```python
from build123d import *

# Parameters (mm, degrees)
SKETCH_1_R          = 2.5
EXTRUDE_1_DEPTH     = 10
SKETCH_2_R          = 2.5
CUT_EXTRUDE_1_DEPTH = 5
SKETCH_3_R          = 2.5
CUT_EXTRUDE_2_DEPTH = 5


with BuildPart() as part:
    # 草图1 → 凸台-拉伸1 (new body)
    with BuildSketch(Plane.XY):
        with BuildLine():
            Line((5, 0), (15, 0))
            Line((15, 0), (15, -5))
            Line((15, -5), (-15, -5))
            Line((-15, -5), (-15, 0))
            Line((-15, 0), (-5, 0))
            Line((-5, 0), (-5, 6))
            ThreePointArc((-5, 6), (0, 11), (5, 6))
            Line((5, 6), (5, 0))
        make_face()
        with Locations((0, 6)):
            Circle(SKETCH_1_R, mode=Mode.SUBTRACT)
    extrude(amount=EXTRUDE_1_DEPTH)

    # 草图2 → 切除-拉伸1 (cut)
    with BuildSketch(Plane(origin=(0, 0, 0), x_dir=(1, 0, 0), z_dir=(0, 1, 0))):
        with Locations(Location((-10, -5, 0), (0, 0, 180))):
            Circle(SKETCH_2_R)
    extrude(amount=-CUT_EXTRUDE_1_DEPTH, mode=Mode.SUBTRACT)

    # 草图3 → 切除-拉伸2 (cut)
    with BuildSketch(Plane(origin=(0, 0, 0), x_dir=(1, 0, 0), z_dir=(0, 1, 0))):
        with Locations(Location((10, -5, 0), (0, 0, 180))):
            Circle(SKETCH_3_R)
    extrude(amount=-CUT_EXTRUDE_2_DEPTH, mode=Mode.SUBTRACT)


solid = part.part
```
The model under review builds one solid part; all positions refer to its coordinate system, in mm. A direction names the side the tool comes from. Coordinates: 2 decimals unless noted, no trailing zeros. Write each loop counter-clockwise with the first axis right and the second up, starting at its lowest first coordinate (ties: lowest second). Pieces come first, ordered by that corner, then holes.
1) To check wall thickness, follow probe 1 along Z at (x, y) = (-10, -2.5); probe 2 along X at (y, z) = (-0.5, 4); probe 3 along Y at (x, z) = (0, 6.5). State the ranges of each line that lie inside material, in increasing order.
2) We need section D-D on y = 6.5. State the section outline as (x, z) points.
3) Clearance check with flat-ended pins moving along their axes: pin 1 Ø5 at (x, z) = (-12, 6) entering from +Y; pin 2 Ø1.8 at (y, z) = (3.5, 5) entering from +X; pin 3 Ø3 at (x, y) = (0, 6) entering from +Z. State where each tip first meets the part, or that it passes through.
4) We need section C-C on z = 1.75. State the section outline as (x, y) points.
5) We need section A-A on z = 3. State the section outline as (x, y) points.
6) We need section B-B on x = -10. State the section outline as (y, z) points, then the cut area to 3 significant figures.
7) Machinability: for faces 1 (the face through (-5, 3, 5)), 2 (the face through (-0.33, 8.48, 4.93)), which of the approach directions +Z, -Z, +X, -X, +Y, -Y give a long, thin tool a straight path to every point of the face, cutting with its end or side? Answer none if there is none.
8) The part is to be moulded in two halves that separate along X. For faces 3 (the face through (-9.67, -2.46, 7.48)), 4 (the face through (8, 0, 3)), 5 (the face through (5, 3, 5)), say which applies: pulls with the +X half, pulls with the -X half, needs draft (parallel to the pull), parting line crosses it, or undercut.
Answer list:
1. probe 1: z = 0 to 2.5, 7.5 to 10
1. probe 2: x = -15 to -12.29, -7.71 to 7.71, 12.29 to 15
1. probe 3: y = -5 to 3.5, 8.5 to 11
2. outline: (-4.97, 0) - (-2.45, 0) - (-2.45, 10) - (-4.97, 10) - close; (2.45, 0) - (4.97, 0) - (4.97, 10) - (2.45, 10) - close
3. pin 1: stops at y = 0
3. pin 2: stops at x = 5
3. pin 3: passes through
4. outline: (-15, -5) - (15, -5) - (15, 0) - (5, 0) - (5, 6) arc R5 ccw to (-5, 6) - (-5, 0) - (-15, 0) - close; hole circle Ø5 at (0, 6)
5. outline: (-15, -5) - (-11.5, -5) - (-11.5, 0) - (-15, 0) - close; (-8.5, -5) - (8.5, -5) - (8.5, 0) - (5, 0) - (5, 6) arc R5 ccw to (-5, 6) - (-5, 0) - (-8.5, 0) - close; (11.5, -5) - (15, -5) - (15, 0) - (11.5, 0) - close; hole circle Ø5 at (0, 6)
6. outline: (-5, 0) - (0, 0) - (0, 2.5) - (-5, 2.5) - close; (-5, 7.5) - (0, 7.5) - (0, 10) - (-5, 10) - close
6. area: 25.0 mm2
7. face 1: +Z, -Z, -X, +Y
7. face 2: +Z, -Z
8. face 3: undercut
8. face 4: needs draft
8. face 5: pulls with the +X half
